Can you work these out from the model? Positions are in its coordinate system, mm. Coordinates: 2 decimals unless noted, no trailing zeros. Use one line per item in the form item = value. Start each with the question number.
(1) If we section it at A-A on z = 1.5: Give the number of separate pieces and of enclosed holes in the cut face, then the cut area to 3 significant figures.
(2) Thinking about a two-plate mould opening in Y: for faces 1 (the face through (53.1, -64.2, 4.8)), 2 (the face through (-9, 60.971, 5)), 3 (the face through (37.53, -54.42, 4.7)), which applies, pulls with the +Y half, pulls with the -Y half, needs draft (parallel to the pull), parting line crosses it, or undercut?
(3) If I drill on probe 1 along X at (y, z) = (49, 3.75); probe 2 along Y at (x, z) = (-62, 3); probe 3 along Y at (x, z) = (44, 2), over which ranges is the centre line in solid material (lowest first)? Write a range as from..to.
```python
from build123d import *

# Parameters (mm, degrees)
F0_W     = 127
F0_H     = 127
F0_R     = 4.7625
F1_DEPTH = 9.525
F2_R     = 6.35


with BuildPart() as f1:
    # F0 (on Top) → F1 (new body)
    with BuildSketch(Plane.XY):
        with Locations((-8.511175, -2.529345)):
            Rectangle(F0_W, F0_H)
        with Locations((-59.311175, -51.588815)):
            Circle(F0_R, mode=Mode.SUBTRACT)
        with Locations((42.288825, -54.632434)):
            Circle(F0_R, mode=Mode.SUBTRACT)
        with Locations((-59.311175, 48.270655)):
            Circle(F0_R, mode=Mode.SUBTRACT)
        with Locations((42.288825, 46.967566)):
            Circle(F0_R, mode=Mode.SUBTRACT)
    extrude(amount=F1_DEPTH)

    # F2
    f2_edges = [f1.edges().sort_by_distance(p)[0] for p in [
        (-72.011175, -66.029345, 4.7625),
        (54.988825, -66.029345, 4.7625),
        (-72.011175, 60.970655, 4.7625),
        (54.988825, 60.970655, 4.7625),
    ]]
    fillet(f2_edges, radius=F2_R)


solid = f1.part
```
Reported:
q1.separate_pieces = 1
q1.enclosed_holes = 4
q1.area = 15,800 mm2
q2.face_1 = pulls with the -Y half
q2.face_2 = pulls with the +Y half
q2.face_3 = undercut
q3.probe_1 = -72.01..-64.02, -54.6..37.98, 46.6..54.99
q3.probe_2 = -66.03..-55.52, -47.66..44.34, 52.2..60.97
q3.probe_3 = -66.03..-59.08, -50.19..42.52, 51.41..60.97
